Read the model definition and answer for the solid it produces. Units are mm, in the model's axes. Face numbers are marked on the shaded views. A direction names the side the tool comes from. Give positions to 0.01 mm unless a question says otherwise; leave off trailing zeros. Order: outer loops, then holes, each group sorted by start corner. A loop starts at its lowest first (then second) coordinate and runs counter-clockwise, first axis right, second up. Notation, with made-up numbers: (28.5, -6) - (86.5, -6) arc R10 cw to (86.5, 9) - close; hole circle Ø4 at (8, -15.75). An arc over 180 degrees is marked (long way). Return JSON: item names as keys, results as strings.
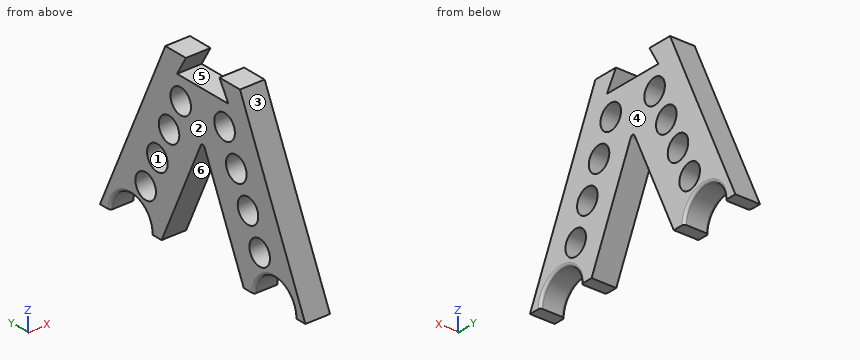
```python
from build123d import *

# Parameters (mm, degrees)
F0_R     = 6.35
F1_DEPTH = 12.7
F3_R     = 1.27


with BuildPart() as f1:
    # F0 (on Right) → F1 (new body)
    with BuildSketch(Plane.YZ):
        with BuildLine():
            Line((-23.075738686, 88.9), (-63.5, 0))
            Line((-63.5, 0), (-57.15, 0))
            ThreePointArc((-57.15, 0), (-44.45, 12.7), (-31.75, 0))
            Line((-31.75, 0), (-25.4, 0))
            Line((-25.4, 0), (0, 55.85902937))
            Line((0, 55.85902937), (0, 79.375))
            Line((0, 79.375), (-15.875, 79.375))
            Line((-15.875, 79.375), (-10.375738686, 88.9))
            Line((-10.375738686, 88.9), (-23.075738686, 88.9))
        make_face()
        with Locations((-35.2503683902, 20.2315941844)):
            Circle(F0_R, mode=Mode.SUBTRACT)
        with Locations((-28.0220864111, 36.1278467579)):
            Circle(F0_R, mode=Mode.SUBTRACT)
        with Locations((-20.7938044319, 52.0240993314)):
            Circle(F0_R, mode=Mode.SUBTRACT)
        with Locations((-13.5655224528, 67.9203519049)):
            Circle(F0_R, mode=Mode.SUBTRACT)
    extrude(amount=F1_DEPTH)

    # F2: F1 across plane


with BuildPart() as f1_1:
    add(f1.part)
    add(f1.part.mirror(Plane.XZ))

    # F3
    f3_edges = [f1_1.edges().sort_by_distance(p)[0] for p in [
        (12.7, 44.45, 12.7),
        (0, 44.45, 12.7),
        (0, -44.45, 12.7),
        (12.7, -44.45, 12.7),
        (6.35, 0, 55.859029),
    ]]
    fillet(f3_edges, radius=F3_R)


solid = f1_1.part
```
Q1. A cutting plane is placed at C-C (x = 8.5). Give the number of separate pieces and of enclosed holes in the cut face, and give its area (3 significant figures).
Values:
{"separate pieces": "1", "enclosed holes": "8", "area": "4,510 mm²"}
Q2. A cutting plane is placed at B-B (z = 41). Write down the section's boundary in (x, y), and give its area (3 significant figures).
Values:
{"outline": "(0, -44.86) - (12.7, -44.86) - (12.7, -32.09) - (0, -32.09) - close; (0, -23.95) - (12.7, -23.95) - (12.7, -6.76) - (0, -6.76) - close; (0, 6.76) - (12.7, 6.76) - (12.7, 23.95) - (0, 23.95) - close; (0, 32.09) - (12.7, 32.09) - (12.7, 44.86) - (0, 44.86) - close", "area": "761 mm²"}
Q3. Determine the mould class of the marked faces 1, 2 and 3 for opening direction Y: released by +Y, released by -Y, zero draft, split by the parting line, or undercut.
Values:
{"face 1": "undercut", "face 2": "zero draft", "face 3": "released by -Y"}
Q4. For the marked faces 4, 5 and 6, determine the directions among +Z, -Z, +X, -X, +Y, -Y from which every point of the face is accessible in a straight line to the end or side of a thin tool.
Values:
{"face 4": "+Z, -Z, +X, +Y, -Y", "face 5": "+X, -X", "face 6": "-Z, +X, -X"}
Q5. Consider L1, parallel to Y at x = 7.75, z = 35; L2, parallel to Y at x = 0.5, z = 10; L3, parallel to Z at x = 5, y = -24. Determine where each line is inside the solid, lowest interval first.
Values:
{"L1": "y = -47.58 to -34.27, -21.77 to -9.48, 9.48 to 21.77, 34.27 to 47.58", "L2": "y = -58.95 to -52.69, -36.21 to -20.85, 20.85 to 36.21, 52.69 to 58.95", "L3": "z = 3.08 to 31.21, 41.04 to 46.54, 57.51 to 86.87"}
Q6. A cutting plane is placed at A-A (z = 83.5). Write down the section's boundary in (x, y).
Values:
{"outline": "(0, -25.53) - (12.7, -25.53) - (12.7, -13.49) - (0, -13.49) - close; (0, 13.49) - (12.7, 13.49) - (12.7, 25.53) - (0, 25.53) - close"}
Q7. Given pin 1 (7.5 mm diameter, centred on y = 20.79, z = 52.02, fed in from +X); pin 2 (3 mm diameter, centred on x = 4.5, z = 38, fed in from -Y); pin 3 (6 mm diameter, centred on x = 4.5, y = -3, fed in from +Z) (3 decimals), each flat-ended and moving along its own axis, determine where each tip first touches the part or whether it passes through.
Values:
{"pin 1": "passes through", "pin 2": "stops at y = -46.9", "pin 3": "stops at z = 79.375"}
Q8. A cutting plane is placed at D-D (y = -44.45). Write down the section's boundary in (x, z), and give its area (3 significant figures).
Values:
{"outline": "(0, 13.97) arc R1.27 ccw to (1.27, 12.7) - (11.43, 12.7) arc R1.27 ccw to (12.7, 13.97) - (12.7, 41.89) - (0, 41.89) - close", "area": "370 mm²"}
